Work out the finished part from the listing and answer in its coordinate system (mm). Face numbers are marked on the shaded views. A direction names the side the tool comes from. Round coordinates to 2 decimals unless told otherwise and drop trailing zeros. Write each loop counter-clockwise with the first axis right and the second up, starting at its lowest first coordinate (ties: lowest second). Pieces come first, ordered by that corner, then holes. Notation, with made-up numbers: (51, 79.25) -> (108, 79.25) arc R36 ccw to (108, 115.25) -> close; hole circle Ø6 at (49, 3). An arc over 180 degrees is marked (long way). Answer as a JSON object with one key per item and string values. Group by question number.
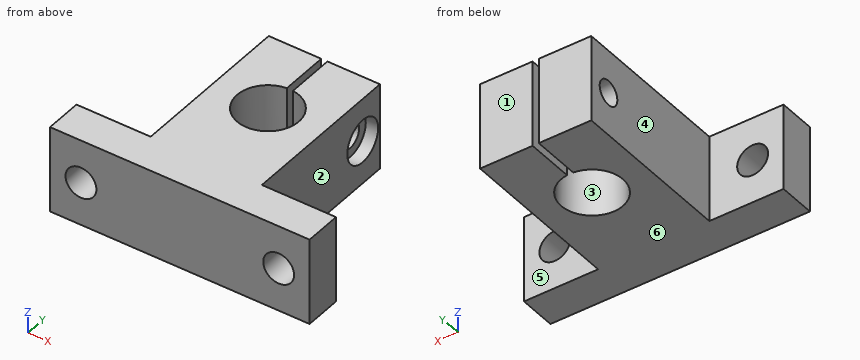
from build123d import *

# Parameters (mm, degrees)
SKETCH_1_R          = 5
EXTRUDE_1_DEPTH     = 14
SKETCH_2_R          = 2.5
CUT_EXTRUDE_1_DEPTH = 7
SKETCH_3_W          = 1
SKETCH_3_H          = 14
CUT_EXTRUDE_2_DEPTH = 14
SKETCH_4_R          = 2
CUT_EXTRUDE_3_DEPTH = 10
SKETCH_5_R          = 3.5
CUT_EXTRUDE_4_DEPTH = 2


with BuildPart() as part:
    # 草图1 → 凸台-拉伸1 (new body)
    with BuildSketch(Plane.XY):
        Polygon((21, 0), (-21, 0), (-21, 6), (-9, 6), (-9, 32.8), (9, 32.8), (9, 6), (21, 6), align=None)
        with Locations((0, 20)):
            Circle(SKETCH_1_R, mode=Mode.SUBTRACT)
    extrude(amount=EXTRUDE_1_DEPTH)

    # 草图2 → 切除-拉伸1 (cut, through all)
    with BuildSketch(Plane(origin=(0, 6, 0), x_dir=(1, 0, 0), z_dir=(0, 1, 0))):
        with Locations((-16, -7)):
            Circle(SKETCH_2_R)
        with Locations((16, -7)):
            Circle(SKETCH_2_R)
    extrude(amount=-CUT_EXTRUDE_1_DEPTH, mode=Mode.SUBTRACT)

    # 草图3 → 切除-拉伸2 (cut)
    with BuildSketch(Plane(origin=(0, 32.8, 0), x_dir=(1, 0, 0), z_dir=(0, 1, 0))):
        with Locations((0, -7)):
            Rectangle(SKETCH_3_W, SKETCH_3_H)
    extrude(amount=-CUT_EXTRUDE_2_DEPTH, mode=Mode.SUBTRACT)

    # 草图4 → 切除-拉伸3 (cut, symmetric)
    with BuildSketch(Plane(origin=(-0.5, 0, 0), x_dir=(0, 0, -1), z_dir=(1, 0, 0))):
        with Locations((-7, 28.887468593)):
            Circle(SKETCH_4_R)
    extrude(amount=CUT_EXTRUDE_3_DEPTH, both=True, mode=Mode.SUBTRACT)

    # 草图5 → 切除-拉伸4 (cut)
    with BuildSketch(Plane(origin=(9, 0, 0), x_dir=(0, 0, -1), z_dir=(1, 0, 0))):
        with Locations((-7, 28.887468593)):
            Circle(SKETCH_5_R)
    extrude(amount=-CUT_EXTRUDE_4_DEPTH, mode=Mode.SUBTRACT)


solid = part.part
1) A cutting plane is placed at D-D on y = 11. Determine the outline of the cut face in (x, z).
2) Straight lines are drawn through the part: L1, parallel to X at y = 3.95, z = 7; L2, parallel to X at y = 31, z = 10.25; L3, parallel to Z at x = 17.5, y = 5.5. For each, find the intervals that lie inside material, in ascending order.
3) A cutting plane is placed at B-B on x = 16. Determine the outline of the cut face in (y, z).
4) For a pull along X with two mould halves and no side action, classify the marked faces 1, 2 and 3 as released by +X, released by -X, zero draft, split by the parting line, or undercut.
5) A cutting plane is placed at C-C on y = 20. Determine the outline of the cut face in (x, z), plus the area to 3 significant figures.
6) A tool of negligible diameter and unlimited length cuts with its end or side. For the marked faces 4, 5 and 6, from which of +Z, -Z, +X, -X, +Y, -Y can it reach the whole face along a straight path? Write none if from no direction.
7) A cutting plane is placed at A-A on z = 7. State how many separate pieces and enclosed holes the cut face has, plus the area to 3 significant figures.
8) Each of these flat-tipped pins is pushed along its axis until it touches: P1, Ø6.5, axis at y = 28, z = 7.5, coming from the +X side; P2, Ø3, axis at y = 10, z = 7.5, coming from the -X side; P3, Ø6.5, axis at x = -16, z = 7, coming from the +Y side; P4, Ø4, axis at x = 16, z = 7, coming from the +Y side. Where does it stop, or does it pass through?
Established:
{
 "1": {"outline": "(-9, 0) -> (9, 0) -> (9, 14) -> (-9, 14) -> close"},
 "2": {"L1": "x = -21 to -18.5, -13.5 to 13.5, 18.5 to 21", "L2": "x = -9 to -0.5, 0.5 to 9", "L3": "z = 0 to 5, 9 to 14"},
 "3": {"outline": "(0, 0) -> (6, 0) -> (6, 4.5) -> (0, 4.5) -> close; (0, 9.5) -> (6, 9.5) -> (6, 14) -> (0, 14) -> close"},
 "4": {"face 1": "zero draft", "face 2": "released by +X", "face 3": "undercut"},
 "5": {"outline": "(-9, 0) -> (-5, 0) -> (-5, 14) -> (-9, 14) -> close; (5, 0) -> (9, 0) -> (9, 14) -> (5, 14) -> close", "area": "112 mm²"},
 "6": {"face 4": "+Z, -Z, -X, +Y", "face 5": "+Z, -Z, +X, +Y", "face 6": "-Z, +X, -X, +Y, -Y"},
 "7": {"separate pieces": "5", "enclosed holes": "0", "area": "514 mm²"},
 "8": {"P1": "stops at x = 9", "P2": "stops at x = -9", "P3": "stops at y = 6", "P4": "passes through"}
}
